Check sheet for the modelled part. Datum: model origin and axes. Units: mm. Round coordinates to 2 decimals unless told otherwise and drop trailing zeros. Write each loop counter-clockwise with the first axis right and the second up, starting at its lowest first coordinate (ties: lowest second). Pieces come first, ordered by that corner, then holes. Notation, with made-up numbers: (71, 36.5) -> (90, 36.5) arc R20 ccw to (90, 73.5) -> close; hole circle Ø2 at (86, 18.25). An arc over 180 degrees is marked (long way). One line per item, written item: value. Start each with the question number.
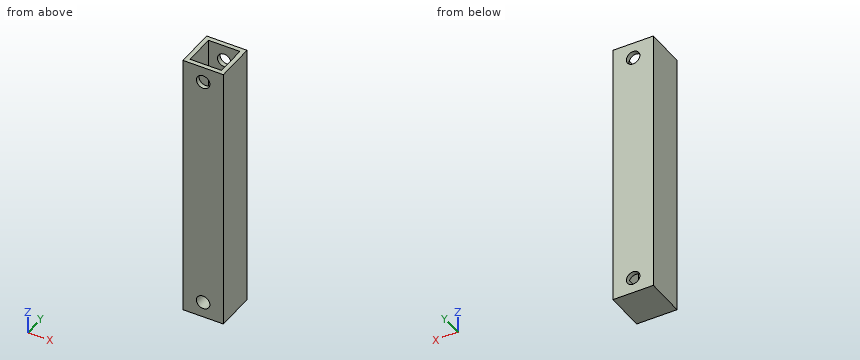
```python
from build123d import *

# Parameters (mm, degrees)
SKETCH_1_W          = 9
SKETCH_1_H          = 9
EXTRUDE_1_DEPTH     = 60
SKETCH_2_W          = 7
SKETCH_2_H          = 7
CUT_EXTRUDE_1_DEPTH = 56
SKETCH_3_R          = 1.5
CUT_EXTRUDE_2_DEPTH = 56


with BuildPart() as part:
    # ｽｹｯﾁ1 → ﾎﾞｽ - 押し出し1 (new body)
    with BuildSketch(Plane.XY):
        Rectangle(SKETCH_1_W, SKETCH_1_H)
    extrude(amount=EXTRUDE_1_DEPTH)

    # ｽｹｯﾁ2 → ｶｯﾄ - 押し出し1 (cut)
    with BuildSketch(Plane.XY.offset(60)):
        Rectangle(SKETCH_2_W, SKETCH_2_H)
    extrude(amount=-CUT_EXTRUDE_1_DEPTH, mode=Mode.SUBTRACT)

    # ｽｹｯﾁ3 → ｶｯﾄ - 押し出し2 (cut)
    with BuildSketch(Plane(origin=(0, 4.5, 0), x_dir=(1, 0, 0), z_dir=(0, 1, 0))):
        with Locations((0, -3.5)):
            Circle(SKETCH_3_R)
        with Locations((0, -56.5)):
            Circle(SKETCH_3_R)
    extrude(amount=-CUT_EXTRUDE_2_DEPTH, mode=Mode.SUBTRACT)


solid = part.part
```
1. Cross-section at D-D (y = 2). Record the cut outline in (x, z), plus the area to 3 significant figures.
2. Depth check by flat-ended pin: pin 1 Ø1.7 at (x, y) = (-2.5, -1.5) entering from +Z; pin 2 Ø3 at (x, y) = (-1, -2.5) entering from -Z. Enter the tip coordinate at first touch or a pass-through.
3. Cross-section at A-A (x = 0). Record the cut outline in (y, z).
4. Cross-section at B-B (z = 3.5). Record the cut outline in (x, y).
5. Material ranges on probe 1 along Z at (x, y) = (0, 3.8); probe 2 along X at (y, z) = (1.25, 45.5), recorded low to high.
6. Cross-section at C-C (x = -2.75). Record the cut outline in (y, z).
Working result:
1. outline: (-4.5, 0) -> (4.5, 0) -> (4.5, 60) -> (3.5, 60) -> (3.5, 4) -> (1.41, 4) arc R1.5 cw (long way) to (-1.41, 4) -> (-3.5, 4) -> (-3.5, 60) -> (-4.5, 60) -> close
1. area: 143 mm^2
2. pin 1: stops at z = 4
2. pin 2: stops at z = 0
3. outline: (-4.5, 0) -> (4.5, 0) -> (4.5, 2) -> (-4.5, 2) -> close; (-4.5, 5) -> (-3.5, 5) -> (-3.5, 55) -> (-4.5, 55) -> close; (-4.5, 58) -> (-3.5, 58) -> (-3.5, 60) -> (-4.5, 60) -> close; (3.5, 5) -> (4.5, 5) -> (4.5, 55) -> (3.5, 55) -> close; (3.5, 58) -> (4.5, 58) -> (4.5, 60) -> (3.5, 60) -> close
4. outline: (-4.5, -4.5) -> (-1.5, -4.5) -> (-1.5, 4.5) -> (-4.5, 4.5) -> close; (1.5, -4.5) -> (4.5, -4.5) -> (4.5, 4.5) -> (1.5, 4.5) -> close
5. probe 1: z = 0 to 2, 5 to 55, 58 to 60
5. probe 2: x = -4.5 to -3.5, 3.5 to 4.5
6. outline: (-4.5, 0) -> (4.5, 0) -> (4.5, 60) -> (3.5, 60) -> (3.5, 4) -> (-3.5, 4) -> (-3.5, 60) -> (-4.5, 60) -> close
